Autodesk Inventor part; units mm, degrees
ref_plane "YZ Plane" through (0, 0, 0) normal (1, 0, 0) x (0, 1, 0)
ref_plane "XZ Plane" through (0, 0, 0) normal (0, 1, 0) x (-1, 0, 0)
ref_plane "XY Plane" through (0, 0, 0) normal (0, 0, 1) x (1, 0, 0)
sketch "草图1" plane through (0, 0, 0) normal (0, 1, 0) x (-1, 0, 0)
  line L0 (18.0685, 16.7445) -> (-61.9315, 16.7445)
  line L1 (-61.9315, 16.7445) -> (-61.9315, -63.2555)
  line L2 (-61.9315, -63.2555) -> (18.0685, -63.2555)
  line L3 (18.0685, -63.2555) -> (18.0685, 16.7445)
  point P0 (0, 0)
  dimension "d0" = 80
  dimension "d1" = 80
extrude "拉伸1" add sketch "草图1" along normal blind 5
sketch "草图2" plane through (0, 5, 0) normal (0, 1, 0) x (1, 0, 0)
  circle A0 centre (46.9315, -1.7445) radius 1.5
  line L0 (61.9315, -16.7445) -> (61.9315, 63.2555)
  line L1 (-18.0685, -16.7445) -> (61.9315, -16.7445)
  circle A1 centre (-3.0685, -1.7445) radius 1.5
  circle A2 centre (-3.0685, 48.2555) radius 1.5
  circle A3 centre (46.9315, 48.2555) radius 1.5
  point P0 (0, 0)
  dimension "d4" = 15
  dimension "d5" = 15
  dimension "d6" = 3
  dimension "d9" = 50
  dimension "d16" = 50
  dimension "d23" = 50
extrude "拉伸2" cut sketch "草图2" against normal blind 5
sketch "草图3" plane through (61.9315, 0, 16.7445) normal (1, 0, 0) x (0, 0, -1)
  line L0 (0, 38) -> (80, 38)
  line L1 (80, 38) -> (80, 0)
  line L2 (80, 0) -> (0, 0)
  line L3 (0, 0) -> (0, 38)
  line L4 (0, 0) -> (80, 0)
  line L5 (0, 0) -> (0, 5)
  point P0 (16.7445, 0)
  point P1 (0, 2.5)
  point P2 (0, 19)
  dimension "d30" = 38
  dimension "d31" = 80
  dimension "d32" = 0
  dimension "d33" = 0
extrude "拉伸3" add sketch "草图3" along normal blind 5
sketch "草图4" plane through (66.9315, 0, 16.7445) normal (1, 0, 0) x (0, 0, -1)
  circle A0 centre (40, 19) radius 14
  line L0 (0, 38) -> (0, 0)
  line L1 (0, 0) -> (80, 0)
  point P0 (16.7445, 0)
  point P1 (40, 0)
  dimension "d36" = 28
  dimension "d37" = 40
  dimension "d38" = 19
extrude "拉伸4" cut sketch "草图4" against normal blind 5
properties part number "电机底座"
The model under review builds one solid part; all positions refer to its coordinate system, in mm. A direction names the side the tool comes from. Coordinates: 2 decimals unless noted, no trailing zeros. Write each loop counter-clockwise with the first axis right and the second up, starting at its lowest first coordinate (ties: lowest second). Pieces come first, ordered by that corner, then holes. Notation, with made-up numbers: (32.25, 80) - (51.25, 80) arc R14 ccw to (51.25, 107) - close; hole circle Ø3 at (58.25, -32). An arc over 180 degrees is marked (long way). Answer in a Markdown table with one row per item. Add a question column.
Q1. To check wall thickness, follow line 1 along Z through (x, y) = (62.95, 19); line 2 along Y through (x, z) = (17, -3); line 3 along X through (y, z) = (24, -46). State the ranges of each line that lie inside material, in increasing order. Write a range as from..to.
Q2. Consider section D-D on x = 35. Give the boundary of the cut face in (y, z), then the cut area to 3 significant figures.
Q3. Clearance check with flat-ended pins moving along their axes: pin 1 (6 mm diameter, centred on x = 22.5, z = -16.5, fed in from +Y); pin 2 (3 mm diameter, centred on y = 16.5, z = -50, fed in from -X); pin 3 (2.5 mm diameter, centred on x = -3.07, z = 1.74, fed in from -Y). State where each tip first meets the part, or that it passes through.
Q4. Consider section B-B on z = -27.5. Give the boundary of the cut face in (x, y).
Q5. For faces 1 (the face through (-1.64, 2.54, 1.29)), 2 (the face through (22, 5, -23)), list the 3-axis set-ups (+Z, -Z, +X, -X, +Y, -Y) from which the entire face can be reached by the end or side of a thin tool; tool diameter is ignored.
Q6. Draft analysis for pull direction X (two halves, no side actions). For faces 3 (the face through (-3.264, 2.535, -49.743)), 4 (the face through (40, 4, -63.256)), 5 (the face through (61.932, 33, -14)), state which applies: +X half, -X half, draft (parallel to the pull), parting line (faces both ways), or undercut.
Q7. Consider section A-A on y = 19. Give the boundary of the cut face in (x, z).
Q8. Consider section C-C on z = -5. Give the boundary of the cut face in (x, y), then the cut area to 3 significant figures.
Answers below:
| question | item | result |
|---|---|---|
| 1 | line 1 | -63.26..-37.26, -9.26..16.74 |
| 1 | line 2 | 0..5 |
| 1 | line 3 | 61.93..66.93 |
| 2 | outline | (0, -63.26) - (5, -63.26) - (5, 16.74) - (0, 16.74) - close |
| 2 | area | 400 mm² |
| 3 | pin 1 | y = 5 |
| 3 | pin 2 | x = 61.93 |
| 3 | pin 3 | through |
| 4 | outline | (-18.07, 0) - (66.93, 0) - (66.93, 5.66) - (61.93, 5.66) - (61.93, 5) - (-18.07, 5) - close; (61.93, 32.34) - (66.93, 32.34) - (66.93, 38) - (61.93, 38) - close |
| 5 | face 1 | +Y, -Y |
| 5 | face 2 | +Z, -Z, -X, +Y |
| 6 | face 3 | undercut |
| 6 | face 4 | draft |
| 6 | face 5 | -X half |
| 7 | outline | (61.93, -63.26) - (66.93, -63.26) - (66.93, -37.26) - (61.93, -37.26) - close; (61.93, -9.26) - (66.93, -9.26) - (66.93, 16.74) - (61.93, 16.74) - close |
| 8 | outline | (-18.07, 0) - (66.93, 0) - (66.93, 38) - (61.93, 38) - (61.93, 5) - (-18.07, 5) - close |
| 8 | area | 590 mm² |
